Input: part model. Units: mm. Frame: model coordinates. A direction names the side the tool comes from. Give positions to 0.01 mm unless a question says otherwise; leave off trailing zeros. Loops run counter-clockwise (first coordinate to the right, second up) from the corner with the lowest first, then second, coordinate; pieces in that order, holes last. Notation, with made-up numbers: (-14.5, 67.5) - (3.5, 67.5) arc R31 ccw to (3.5, 95.5) - close; hole circle Ø7 at (-8, 83). An arc over 180 degrees is marked (long way). Answer as a JSON object with one key per item and string values.
from build123d import *

# Parameters (mm, degrees)
F0_R      = 12.45
F1_DEPTH  = 12
F2_R      = 14.5
F3_DEPTH  = 3
F4_R      = 9.95
F5_DEPTH  = 70
F7_DEPTH  = 20
F10_DEPTH = 25
F11_R     = 0.5


with BuildPart() as f1:
    # F0 (on Front) → F1 (new body)
    with BuildSketch(Plane.XZ):
        Circle(F0_R)
    extrude(amount=-F1_DEPTH)

    # F2 (on Front) → F3 (join)
    with BuildSketch(Plane.XZ):
        Circle(F2_R)
    extrude(amount=F3_DEPTH)

    # F4 (on face) → F5 (join)
    with BuildSketch(Plane.XZ.offset(3)):
        Circle(F4_R)
    extrude(amount=F5_DEPTH)

    # F6 (on face) → F7 (join)
    with BuildSketch(Plane.XZ.offset(3)):
        with BuildLine():
            Line((2, 9.7469225913), (2, 12.3389626793))
            ThreePointArc((2, 12.3389626793), (0, 12.5), (-2, 12.3389626793))
            Line((-2, 12.3389626793), (-2, 9.7469225913))
            ThreePointArc((-2, 9.7469225913), (0, 9.95), (2, 9.7469225913))
        make_face()
        with BuildLine():
            Line((5.6346263027, 11.1580010051), (4.1110633656, 9.0609965238))
            ThreePointArc((4.1110633656, 9.0609965238), (5.8484632603, 8.049719094), (7.3471313431, 6.7098555146))
            Line((7.3471313431, 6.7098555146), (8.8706942802, 8.8068599959))
            ThreePointArc((8.8706942802, 8.8068599959), (7.3473156537, 10.1127124297), (5.6346263027, 11.1580010051))
        make_face()
        with BuildLine():
            Line((11.1170168717, 5.7150621934), (8.6518402555, 4.9140777561))
            ThreePointArc((8.6518402555, 4.9140777561), (9.4630123371, 3.074719094), (9.887908233, 1.109851691))
            Line((9.887908233, 1.109851691), (12.3530848492, 1.9108361283))
            ThreePointArc((12.3530848492, 1.9108361283), (11.8882064537, 3.8627124297), (11.1170168717, 5.7150621934))
        make_face()
        with BuildLine():
            Line((12.3530848492, -1.9108361283), (9.887908233, -1.109851691))
            ThreePointArc((9.887908233, -1.109851691), (9.4630123371, -3.074719094), (8.6518402555, -4.9140777561))
            Line((8.6518402555, -4.9140777561), (11.1170168717, -5.7150621934))
            ThreePointArc((11.1170168717, -5.7150621934), (11.8882064537, -3.8627124297), (12.3530848492, -1.9108361283))
        make_face()
        with BuildLine():
            Line((8.8706942802, -8.8068599959), (7.3471313431, -6.7098555146))
            ThreePointArc((7.3471313431, -6.7098555146), (5.8484632603, -8.049719094), (4.1110633656, -9.0609965238))
            Line((4.1110633656, -9.0609965238), (5.6346263027, -11.1580010051))
            ThreePointArc((5.6346263027, -11.1580010051), (7.3473156537, -10.1127124297), (8.8706942802, -8.8068599959))
        make_face()
        with BuildLine():
            ThreePointArc((2, -9.7469225913), (0, -9.95), (-2, -9.7469225913))
            Line((-2, -9.7469225913), (-2, -12.3389626793))
            ThreePointArc((-2, -12.3389626793), (0, -12.5), (2, -12.3389626793))
            Line((2, -12.3389626793), (2, -9.7469225913))
        make_face()
        with BuildLine():
            ThreePointArc((-4.1110633656, -9.0609965238), (-5.8484632603, -8.049719094), (-7.3471313431, -6.7098555146))
            Line((-7.3471313431, -6.7098555146), (-8.8706942802, -8.8068599959))
            ThreePointArc((-8.8706942802, -8.8068599959), (-7.3473156537, -10.1127124297), (-5.6346263027, -11.1580010051))
            Line((-5.6346263027, -11.1580010051), (-4.1110633656, -9.0609965238))
        make_face()
        with BuildLine():
            ThreePointArc((-8.6518402555, -4.9140777561), (-9.4630123371, -3.074719094), (-9.887908233, -1.109851691))
            Line((-9.887908233, -1.109851691), (-12.3530848492, -1.9108361283))
            ThreePointArc((-12.3530848492, -1.9108361283), (-11.8882064537, -3.8627124297), (-11.1170168717, -5.7150621934))
            Line((-11.1170168717, -5.7150621934), (-8.6518402555, -4.9140777561))
        make_face()
        with BuildLine():
            ThreePointArc((-9.887908233, 1.109851691), (-9.4630123371, 3.074719094), (-8.6518402555, 4.9140777561))
            Line((-8.6518402555, 4.9140777561), (-11.1170168717, 5.7150621934))
            ThreePointArc((-11.1170168717, 5.7150621934), (-11.8882064537, 3.8627124297), (-12.3530848492, 1.9108361283))
            Line((-12.3530848492, 1.9108361283), (-9.887908233, 1.109851691))
        make_face()
        with BuildLine():
            ThreePointArc((-7.3471313431, 6.7098555146), (-5.8484632603, 8.049719094), (-4.1110633656, 9.0609965238))
            Line((-4.1110633656, 9.0609965238), (-5.6346263027, 11.1580010051))
            ThreePointArc((-5.6346263027, 11.1580010051), (-7.3473156537, 10.1127124297), (-8.8706942802, 8.8068599959))
            Line((-8.8706942802, 8.8068599959), (-7.3471313431, 6.7098555146))
        make_face()
    extrude(amount=F7_DEPTH)

    # F9 (on offset) → F10 (cut)
    with BuildSketch(Plane.XY.offset(6)):
        with BuildLine():
            Line((-3, -53.2881170511), (-3, -79.6965509653))
            Line((-3, -79.6965509653), (3, -79.6965509653))
            Line((3, -79.6965509653), (3, -53.2881170511))
            ThreePointArc((3, -53.2881170511), (0, -50.2881170511), (-3, -53.2881170511))
        make_face()
    extrude(amount=F10_DEPTH, mode=Mode.SUBTRACT)

    # F11
    f11_edges = [f1.edges().sort_by_distance(p)[0] for p in [
        (-3, -63.144059, 9.486965),
        (3, -63.144059, 9.486965),
        (0, -50.288117, 9.95),
    ]]
    fillet(f11_edges, radius=F11_R)


solid = f1.part
Item 1: Material intervals for line 1 (Y direction, x = -11, z = -5.25); line 2 (X direction, y = -22, z = 10.75); line 3 (X direction, y = -12.5, z = 10.25), sorted ascending. Write a range as [from, to].
Geometry check:
{"line 1": "y = [-23, 12]", "line 2": "x = [-6.38, -5.34], [-2, 2], [5.34, 6.38]", "line 3": "x = [-7.15, -4.97], [-2, 2], [4.97, 7.15]"}
Item 2: Cut plane B-B (y = -47). Return loops of the section in (x, z), then the cut area to 3 significant figures.
Geometry check:
{"outline": "circle Ø19.9 at (0, 0)", "area": "311 mm2"}
Item 3: Mould query, pull axis X, two halves, no side actions, for faces 1 (the face through (0, -61, 6)), 2 (the face through (7.325, -12.86, -10.129)), 3 (the face through (-11.103, -12.86, -1.505)). Classes: released by +X, released by -X, zero draft, split by the parting line, or undercut.
Geometry check:
{"face 1": "undercut", "face 2": "released by +X", "face 3": "released by -X"}
Item 4: Cut plane D-D (y = -59.5). Return loops of the section in (x, z), then the cut area to 3 significant figures.
Geometry check:
{"outline": "(-3.69, 9.24) arc R9.95 ccw (long way) to (3.69, 9.24) arc R0.5 ccw to (3, 8.78) - (3, 6) - (-3, 6) - (-3, 8.78) arc R0.5 ccw to start", "area": "288 mm2"}
Item 5: Contact query for flat-ended pins moving along their axis: P1, Ø1.4, axis at x = -1, z = -10.5, coming from the -Y side; P2, Ø6, axis at x = -10.5, y = -43.5, coming from the -Z side; P3, Ø0.8, axis at y = -63.5, z = 7.5, coming from the +X side; P4, Ø3.5, axis at x = 7, z = -9.5, coming from the -Y side. Output: stop coordinate, or through.
Geometry check:
{"P1": "stops at y = -73", "P2": "stops at z = -6.54", "P3": "stops at x = 6.97", "P4": "stops at y = -23"}
Item 6: Access query for faces 4 (the face through (11.103, -12.86, 1.505)), 5 (the face through (-4.88, -12.86, -10.12)), 6 (the face through (-4.86, -12.86, 10.09)), 7 (the face through (-7.37, -12.86, -10.096)). Directions: +Z, -Z, +X, -X, +Y, -Y. A direction counts if a zero-diameter tool reaches every point of the face in a straight line with its end or side. Return the directions, or none.
Geometry check:
{"face 4": "+X, -Y", "face 5": "-Z, -Y", "face 6": "+Z, -Y", "face 7": "-Z, -X, -Y"}
Item 7: Cut plane A-A (z = 0). Return loops of the section in (x, y), then the cut area to 3 significant figures.
Geometry check:
{"outline": "(-14.5, -3) - (-9.95, -3) - (-9.95, -73) - (9.95, -73) - (9.95, -3) - (14.5, -3) - (14.5, 0) - (12.45, 0) - (12.45, 12) - (-12.45, 12) - (-12.45, 0) - (-14.5, 0) - close", "area": "1,780 mm2"}
Item 8: Cut plane C-C (y = 6.5). Return loops of the section in (x, z).
Geometry check:
{"outline": "circle Ø24.9 at (0, 0)"}
